Here's the drawing with two shaded views (mm, measured from the low corner). I have some questions. Give positions to 0.01 mm unless a question says otherwise; leave off trailing zeros. Loops run counter-clockwise (first coordinate to the right, second up) from the corner with the lowest first, then second, coordinate; pieces in that order, holes last. Notation, with made-up numbers: (28, 80) - (49, 80) arc R15 cw to (49, 105) - close; hole circle Ø11 at (-6.5, 51). An arc over 180 degrees is marked (long way). Write each question's results on one line, items separated by ' | '. Start each with the question number.
1) If we mould it in two halves opening along Y, with no side actions, what happens to the marked faces 1 and 2? For each: +Y half, -Y half, draft (parallel to the pull), parting line (faces both ways), or undercut.
2) I want a section at A-A, the plane y = 6.35. Write out the boundary of the cut face in (x, z), and give its area (3 significant figures).
3) I want a section at C-C, the plane x = 3.5. Write out the boundary of the cut face in (y, z), and give its area (3 significant figures).
4) I want a section at D-D, the plane z = 35.5. Write out the boundary of the cut face in (x, y).
5) I want a section at B-B, the plane x = 6.35. Write out the boundary of the cut face in (y, z) (3 decimals), and give its area (3 significant figures).
6) If I drill on probe 1 along Z at (x, y) = (6.35, 12.1) (3 decimals); probe 2 along Y at (x, z) = (6, 57), over which ranges is the centre line in solid material (lowest first)? Write a range as [from, to].
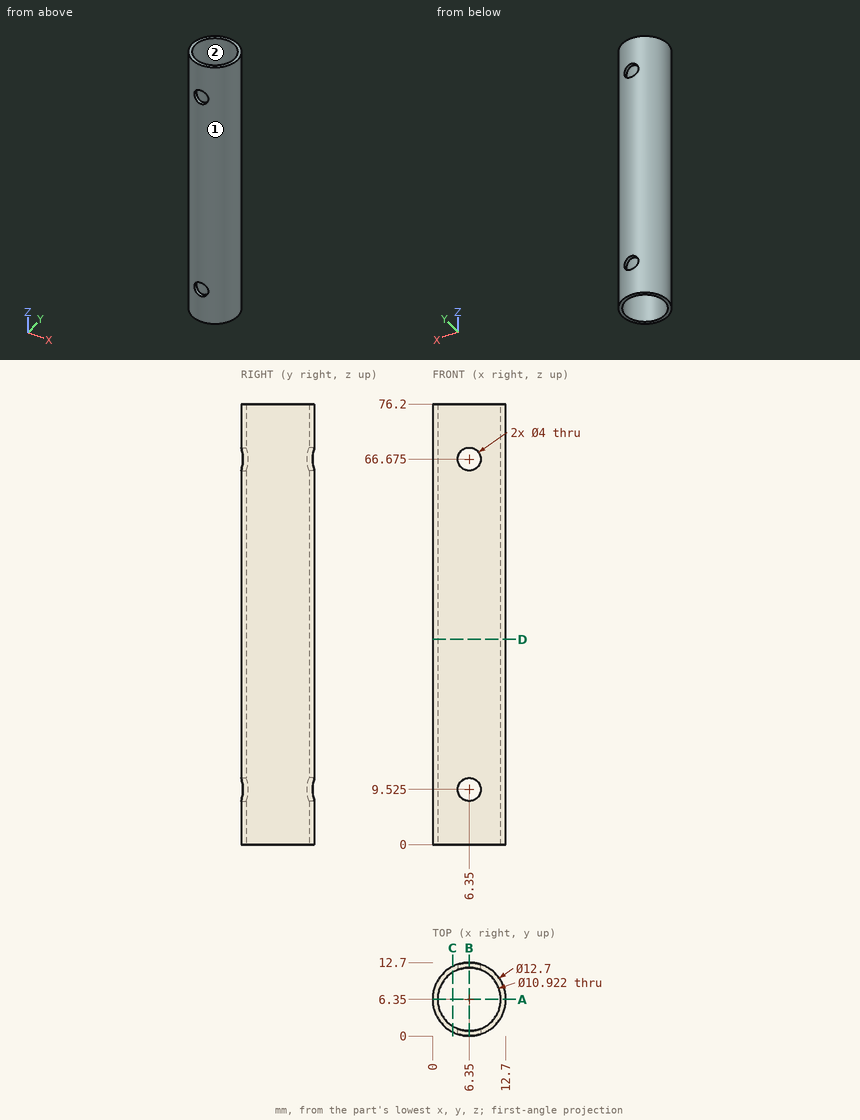
Answers:
1) face 1: parting line | face 2: undercut
2) outline: (0, 0) - (0.89, 0) - (0.89, 76.2) - (0, 76.2) - close; (11.81, 0) - (12.7, 0) - (12.7, 76.2) - (11.81, 76.2) - close | area: 135 mm2
3) outline: (0.68, 0) - (1.69, 0) - (1.69, 76.2) - (0.68, 76.2) - close; (11.01, 0) - (12.02, 0) - (12.02, 76.2) - (11.01, 76.2) - close | area: 155 mm2
4) outline: circle Ø12.7 at (6.35, 6.35); hole circle Ø10.92 at (6.35, 6.35)
5) outline: (0, 0) - (0.889, 0) - (0.889, 7.525) - (0, 7.525) - close; (0, 11.525) - (0.889, 11.525) - (0.889, 64.675) - (0, 64.675) - close; (0, 68.675) - (0.889, 68.675) - (0.889, 76.2) - (0, 76.2) - close; (11.811, 0) - (12.7, 0) - (12.7, 7.525) - (11.811, 7.525) - close; (11.811, 11.525) - (12.7, 11.525) - (12.7, 64.675) - (11.811, 64.675) - close; (11.811, 68.675) - (12.7, 68.675) - (12.7, 76.2) - (11.811, 76.2) - close | area: 121 mm2
6) probe 1: z = [0, 7.525], [11.525, 64.675], [68.675, 76.2] | probe 2: y = [0.01, 0.9], [11.8, 12.69]
